Autodesk Inventor part; units mm, degrees
ref_plane "YZ Plane" through (0, 0, 0) normal (1, 0, 0) x (0, 1, 0)
ref_plane "XZ Plane" through (0, 0, 0) normal (0, 1, 0) x (-1, 0, 0)
ref_plane "XY Plane" through (0, 0, 0) normal (0, 0, 1) x (1, 0, 0)
sketch "Sketch1" plane through (0, 0, 0) normal (0, 1, 0) x (-1, 0, 0)
  line L0 (0, 0) -> (85, 0)
  line L1 (85, 0) -> (85, -160)
  line L2 (85, -160) -> (0, -160)
  line L3 (0, -160) -> (0, 0)
  dimension "d0" = 85
  dimension "d1" = 160
extrude "Extrusion1" add sketch "Sketch1" along normal blind 3
fillet "Fillet1" radius 2 4 edges at (0, 1.5, 0) (-85, 1.5, 0) (-85, 1.5, -160) (0, 1.5, -160)
sketch "Sketch2" plane through (0, 3, 0) normal (0, 1, 0) x (1, 0, 0)
  arc A0 (0, 158) -> (-2, 160) centre (-2, 158) ccw
  line L0 (-2, 160) -> (-83, 160)
  arc A1 (-83, 160) -> (-85, 158) centre (-83, 158) ccw
  line L1 (-85, 158) -> (-85, 2)
  arc A2 (-85, 2) -> (-83, 0) centre (-83, 2) ccw
  line L2 (-83, 0) -> (-2, 0)
  arc A3 (-2, 0) -> (0, 2) centre (-2, 2) ccw
  line L3 (0, 2) -> (0, 158)
  line L4 (-82.5, 2.5) -> (-82.5, 157.5)
  line L5 (-82.5, 157.5) -> (-2.5, 157.5)
  line L6 (-2.5, 157.5) -> (-2.5, 2.5)
  line L7 (-2.5, 2.5) -> (-82.5, 2.5)
  line L8 (-81.75, 156.75) -> (-81.75, 3.25)
  line L9 (-81.75, 3.25) -> (-3.25, 3.25)
  line L10 (-3.25, 3.25) -> (-3.25, 156.75)
  line L11 (-3.25, 156.75) -> (-81.75, 156.75)
  line L12 (-83.25, 158.25) -> (-83.25, 1.75)
  line L13 (-83.25, 1.75) -> (-1.75, 1.75)
  line L14 (-1.75, 1.75) -> (-1.75, 158.25)
  line L15 (-1.75, 158.25) -> (-83.25, 158.25)
  point P0 (0, 0)
  dimension "d5" = 2.5
  dimension "d6" = 0.75
  dimension "d31" = 0.75
extrude "Extrusion2" cut sketch "Sketch2" against normal blind 2 contours L11 L10 L9 L8
extrude "Extrusion3" cut sketch "Sketch2" against normal blind 0.75 contours L15 L14 L13 L12
sketch "Sketch3" plane through (0, 1, 0) normal (0, 1, 0) x (1, 0, 0)
  circle A0 centre (-70, 15) radius 2.5
  circle A1 centre (-15, 15) radius 2.5
  circle A2 centre (-70, 145) radius 2.5
  circle A3 centre (-15, 145) radius 2.5
  circle A4 centre (-70, 15) radius 0.5
  circle A5 centre (-15, 15) radius 0.5
  circle A6 centre (-15, 145) radius 0.5
  circle A7 centre (-70, 145) radius 0.5
  line L0 (-85, 158) -> (-85, 2)
  line L1 (-83, 0) -> (-2, 0)
  line L2 (0, 2) -> (0, 158)
  line L3 (-2, 160) -> (-83, 160)
  point P0 (0, 0)
  dimension "d11" = 5
  dimension "d12" = 5
  dimension "d13" = 5
  dimension "d14" = 5
  dimension "d15" = 2
  dimension "d16" = 2
  dimension "d17" = 2
  dimension "d18" = 2
  dimension "d19" = 15
  dimension "d20" = 15
  dimension "d21" = 15
  dimension "d22" = 15
  dimension "d23" = 15
  dimension "d24" = 15
  dimension "d25" = 15
  dimension "d26" = 15
extrude "Extrusion4" add sketch "Sketch3" along normal blind 1.5 contours A4 | A5 | A6 | A7
extrude "Extrusion5" add sketch "Sketch3" along normal blind 0.5 contours A0 | A1 | A2 | A3 | A4 | A6
sketch "Sketch4" plane through (-2, 0, -160) normal (0, 0, -1) x (-1, 0, 0)
  line L0 (1.25, 3) -> (79.75, 3)
  arc A0 (38.5, 3) -> (42.5, 3) centre (40.5, 3) ccw
  line L1 (0, 0) -> (81, 0)
  line L2 (0, 3) -> (81, 3)
  line L3 (79.75, 1) -> (1.25, 1)
  point P0 (-2, 0)
  point P1 (-2, 3)
  point P2 (40.5, 3)
  point P3 (38.5, 3)
  dimension "d32" = 42.5
  dimension "d33" = 3
extrude "Extrusion6" cut sketch "Sketch4" against normal through all
properties part number "BOTTOM_COVER"
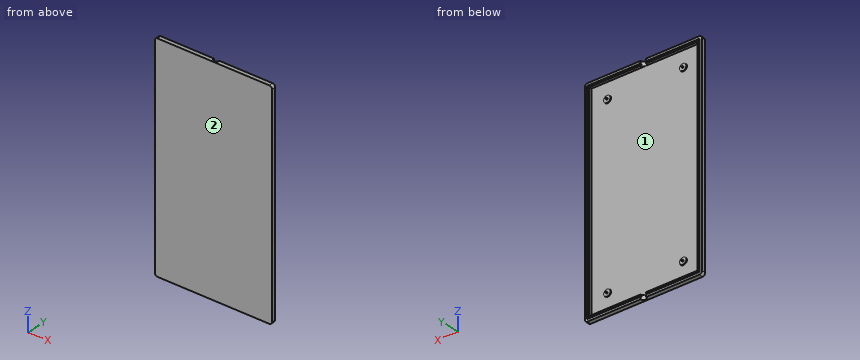
Input: part model. Units: mm. Frame: model coordinates. Face numbers are marked on the shaded views. Give positions to 0.01 mm unless a question says otherwise; leave off trailing zeros. Loops run counter-clockwise (first coordinate to the right, second up) from the corner with the lowest first, then second, coordinate; pieces in that order, holes last.
1) Contact query for flat-ended pins moving along their axis: pin 1 (1.1 mm diameter, centred on x = -15, z = -15, fed in from +Y); pin 2 (10 mm diameter, centred on x = -31.5, z = -102.5, fed in from +Y). Output: stop coordinate, or through.
A:
pin 1: stops at y = 2.5
pin 2: stops at y = 1
2) Line query: L1, parallel to Z at x = -20, y = 2.65; L2, parallel to X at y = 2.55, z = -150.5; L3, parallel to Z at x = -6.5, y = 1.7. Output: solid intervals per line, ascending.
A:
L1: z = -160 to -158.25, -157.5 to -156.75, -3.25 to -2.5, -1.75 to 0
L2: x = -85 to -83.25, -82.5 to -81.75, -3.25 to -2.5, -1.75 to 0
L3: z = -160 to -156.75, -3.25 to 0
3) Section query A-A on z = -41. Return the cut outline in (x, y).
A:
outline: (-85, 0) - (0, 0) - (0, 3) - (-1.75, 3) - (-1.75, 2.25) - (-2.5, 2.25) - (-2.5, 3) - (-3.25, 3) - (-3.25, 1) - (-81.75, 1) - (-81.75, 3) - (-82.5, 3) - (-82.5, 2.25) - (-83.25, 2.25) - (-83.25, 3) - (-85, 3) - close
4) Section query B-B on x = -56. Return the cut outline in (y, z), and give its area (3 significant figures).
A:
outline: (0, -160) - (3, -160) - (3, -158.25) - (2.25, -158.25) - (2.25, -157.5) - (3, -157.5) - (3, -156.75) - (1, -156.75) - (1, -3.25) - (3, -3.25) - (3, -2.5) - (2.25, -2.5) - (2.25, -1.75) - (3, -1.75) - (3, 0) - (0, 0) - close
area: 172 mm2
5) Mould query, pull axis X, two halves, no side actions, for the marked faces 1 and 2. Classes: released by +X, released by -X, zero draft, split by the parting line, or undercut.
A:
face 1: undercut
face 2: zero draft
